Solid Edge part; units mm, degrees
sketch "Sketch1" plane through (0, 0, 0) normal (0, 0, 1) x (1, 0, 0)
  line L0 (41.85, -0.3) -> (0, -0.3)
  line L1 (0, -0.3) -> (0, 0)
  line L2 (0, 0) -> (42.15, 0)
  line L3 (42.15, 0) -> (42.15, -8)
  line L4 (42.15, -8) -> (49.85, -8)
  line L5 (49.85, -8) -> (49.85, -8.3)
  line L6 (49.85, -8.3) -> (41.85, -8.3)
  line L7 (41.85, -8.3) -> (41.85, -0.3)
extrude "ExtrudedProtrusion_1" add sketch "Sketch1" along normal blind 5 and the other way blind 36
sketch "Sketch2" plane through (0, 0, 0) normal (0, -1, 0) x (1, 0, 0)
  circle A0 centre (45.85, 0) radius 1.25
  circle A1 centre (45.85, -32) radius 1.5
extrude "Cutout1" cut sketch "Sketch2" along normal up to next
mirror "Mirror1" about plane through (0, 0, 0) normal (1, 0, 0) of "ExtrudedProtrusion_1", "Cutout1"
sketch "Sketch3" plane through (0, 0, 0) normal (1, 0, 0) x (0, 1, 0)
  line L0 (-15.6936, -26.4307) -> (-0.3, -26.4307)
  line L1 (-0.3, -26.4307) -> (-0.3, -5.4939)
  line L2 (-0.3, -5.4939) -> (-15.6936, -5.4939)
  line L3 (-15.6936, -5.4939) -> (-15.6936, -26.4307)
extrude "Cutout2" cut sketch "Sketch3" against normal up to next
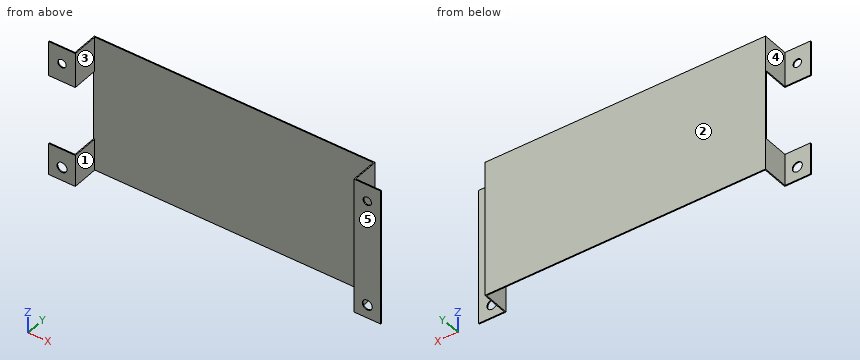
For this review, take the finished solid that the model builds, in its own axes (mm). Face numbers are marked on the shaded views. A direction names the side the tool comes from. Coordinates: 2 decimals unless noted, no trailing zeros. Loops run counter-clockwise (first coordinate to the right, second up) from the corner with the lowest first, then second, coordinate; pieces in that order, holes last. Notation, with made-up numbers: (-38, -22) - (-23, -22) arc R11 ccw to (-23, -4) - close; hole circle Ø2 at (29.5, 68.25). An arc over 180 degrees is marked (long way). Use a Markdown table: item, result. Add a question column.
Item 1: Tool access review of the marked faces 1 and 2: name each direction out of +Z, -Z, +X, -X, +Y, -Y from which nothing blocks a thin tool from reaching the whole face with its end or side.
Item 2: For line 1 (Z direction, x = -45.85, y = -8.15); line 2 (X direction, y = -8.1, z = -32); line 3 (Z direction, x = 45.85, y = -8.15), list the stretches that pass through material, from the lowest coordinate up.
Item 3: We need section A-A (y = -6.25). Give the boundary of the cut face in (x, z), and give its area (3 significant figures).
Item 4: Insertion check: pin 1 Ø5 at (x, z) = (6, -7.5) entering from +Y; pin 2 Ø5 at (x, z) = (45.85, -32) entering from +Y; pin 3 Ø1 at (y, z) = (-4, -30.5) entering from +X; pin 4 Ø3 at (x, z) = (18, -21.5) entering from -Y. Each pin has a flat end and moves straight along its axis. Give the tip position at first contact, or say it passes through.
Item 5: We need section B-B (z = -32). Give the boundary of the cut face in (x, y), and give its area (3 significant figures).
Item 6: We need section D-D (z = 0). Give the boundary of the cut face in (x, y), and give its area (3 significant figures).
Item 7: Mouldability with a two-part tool opening along X and no side actions: class the marked faces 3, 4 and 5 as pulls with the +X half, pulls with the -X half, needs draft (parallel to the pull), parting line crosses it, or undercut.
Item 8: We need section C-C (x = -45.85). Give the boundary of the cut face in (y, z), and give its area (3 significant figures).
Results list:
| question | item | result |
|---|---|---|
| 1 | face 1 | +Z, -Z, -Y |
| 1 | face 2 | +Z, -Z, +X, -X, +Y |
| 2 | line 1 | z = -36 to -33.5, -30.5 to -26.43, -5.49 to -1.25, 1.25 to 5 |
| 2 | line 2 | x = -49.85 to -47.35, -44.35 to -41.85, 41.85 to 44.35, 47.35 to 49.85 |
| 2 | line 3 | z = -36 to -33.5, -30.5 to -1.25, 1.25 to 5 |
| 3 | outline | (-42.15, -36) - (-41.85, -36) - (-41.85, -26.43) - (-42.15, -26.43) - close; (-42.15, -5.49) - (-41.85, -5.49) - (-41.85, 5) - (-42.15, 5) - close; (41.85, -36) - (42.15, -36) - (42.15, 5) - (41.85, 5) - close |
| 3 | area | 18.3 mm^2 |
| 4 | pin 1 | stops at y = 0 |
| 4 | pin 2 | stops at y = -8 |
| 4 | pin 3 | stops at x = 42.15 |
| 4 | pin 4 | stops at y = -0.3 |
| 5 | outline | (-49.85, -8.3) - (-47.35, -8.3) - (-47.35, -8) - (-49.85, -8) - close; (-44.35, -8.3) - (-41.85, -8.3) - (-41.85, -0.3) - (41.85, -0.3) - (41.85, -8.3) - (44.35, -8.3) - (44.35, -8) - (42.15, -8) - (42.15, 0) - (-42.15, 0) - (-42.15, -8) - (-44.35, -8) - close; (47.35, -8.3) - (49.85, -8.3) - (49.85, -8) - (47.35, -8) - close |
| 5 | area | 32.9 mm^2 |
| 6 | outline | (-49.85, -8.3) - (-47.1, -8.3) - (-47.1, -8) - (-49.85, -8) - close; (-44.6, -8.3) - (-41.85, -8.3) - (-41.85, -0.3) - (41.85, -0.3) - (41.85, -8.3) - (44.6, -8.3) - (44.6, -8) - (42.15, -8) - (42.15, 0) - (-42.15, 0) - (-42.15, -8) - (-44.6, -8) - close; (47.1, -8.3) - (49.85, -8.3) - (49.85, -8) - (47.1, -8) - close |
| 6 | area | 33.2 mm^2 |
| 7 | face 3 | undercut |
| 7 | face 4 | pulls with the -X half |
| 7 | face 5 | needs draft |
| 8 | outline | (-8.3, -36) - (-8, -36) - (-8, -33.5) - (-8.3, -33.5) - close; (-8.3, -30.5) - (-8, -30.5) - (-8, -26.43) - (-8.3, -26.43) - close; (-8.3, -5.49) - (-8, -5.49) - (-8, -1.25) - (-8.3, -1.25) - close; (-8.3, 1.25) - (-8, 1.25) - (-8, 5) - (-8.3, 5) - close |
| 8 | area | 4.37 mm^2 |
